Study the drawing (mm; zero at the part's minimum x, y, z) and answer. A direction names the side the tool comes from. Round coordinates to 2 decimals unless told otherwise and drop trailing zeros. Loops run counter-clockwise (first coordinate to the right, second up) from the corner with the lowest first, then second, coordinate; pieces in that order, holes last. Notation, with made-up numbers: (85, -25) -> (124, -25) arc R28 ccw to (124, 4) -> close; hole circle Ø10 at (66, 75.25). An arc over 180 degrees is marked (long way). Use one line per item in the form item = value.
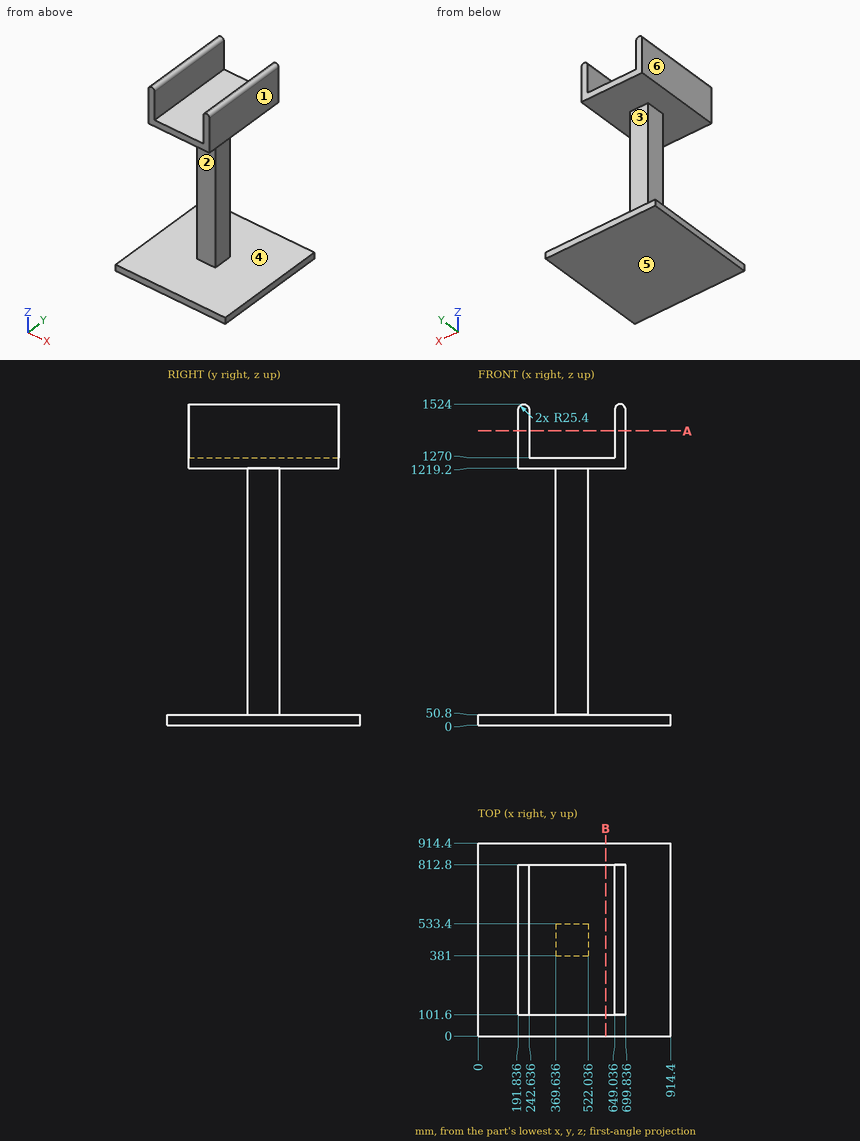
(1) Consider L1, parallel to Z at x = 326.5, y = 520; L2, parallel to X at y = 473.5, z = 501; L3, parallel to Z at x = 67.5, y = 446.5. Determine where each line is inside the solid, lowest interval first.
Completed:
L1 = 0 to 50.8, 1219.2 to 1270
L2 = 369.64 to 522.04
L3 = 0 to 50.8
(2) For the marked faces 1, 2 and 3, determine the directions among +Z, -Z, +X, -X, +Y, -Y from which every point of the face is accessible in a straight line to the end or side of a thin tool.
Completed:
face_1 = +Z, +X, +Y, -Y
face_2 = +X, -X, -Y
face_3 = +X, -X, +Y
(3) For a pull along Z with two mould halves and no side action, classify the marked faces 4, 5 and 6 as +Z half, -Z half, draft (parallel to the pull), parting line (faces both ways), or undercut.
Completed:
face_4 = undercut
face_5 = -Z half
face_6 = draft
(4) Given P1, Ø8, axis at x = 328.5, y = 618, coming from the +Z side; P2, Ø8, axis at y = 423.5, z = 287.5, coming from the -X side, each flat-ended and moving along its own axis, determine where each tip first touches the part or whether it passes through.
Completed:
P1 = 1270
P2 = 369.64
(5) Find section B-B, the plane x = 605. Write down the section's boundary in (y, z).
Completed:
outline = (0, 0) -> (914.4, 0) -> (914.4, 50.8) -> (0, 50.8) -> close; (101.6, 1219.2) -> (812.8, 1219.2) -> (812.8, 1270) -> (101.6, 1270) -> close
(6) Find section A-A, the plane z = 1396. Write down the section's boundary in (x, y), then the cut area to 3 significant figures.
Completed:
outline = (191.84, 101.6) -> (242.64, 101.6) -> (242.64, 812.8) -> (191.84, 812.8) -> close; (649.04, 101.6) -> (699.84, 101.6) -> (699.84, 812.8) -> (649.04, 812.8) -> close
area = 72,300 mm2
